Here's the drawing with two shaded views (mm, measured from the low corner). I have some questions. Round coordinates to 2 decimals unless told otherwise and drop trailing zeros. Order: outer loops, then holes, each group sorted by start corner. A loop starts at its lowest first (then second) coordinate and runs counter-clockwise, first axis right, second up. Notation, with made-up numbers: (56.25, 20) - (75.25, 20) arc R19 cw to (75.25, 26) - close; hole circle Ø3 at (4.25, 25). An arc over 180 degrees is marked (long way). Return JSON: item names as keys, results as strings. Group by question number.
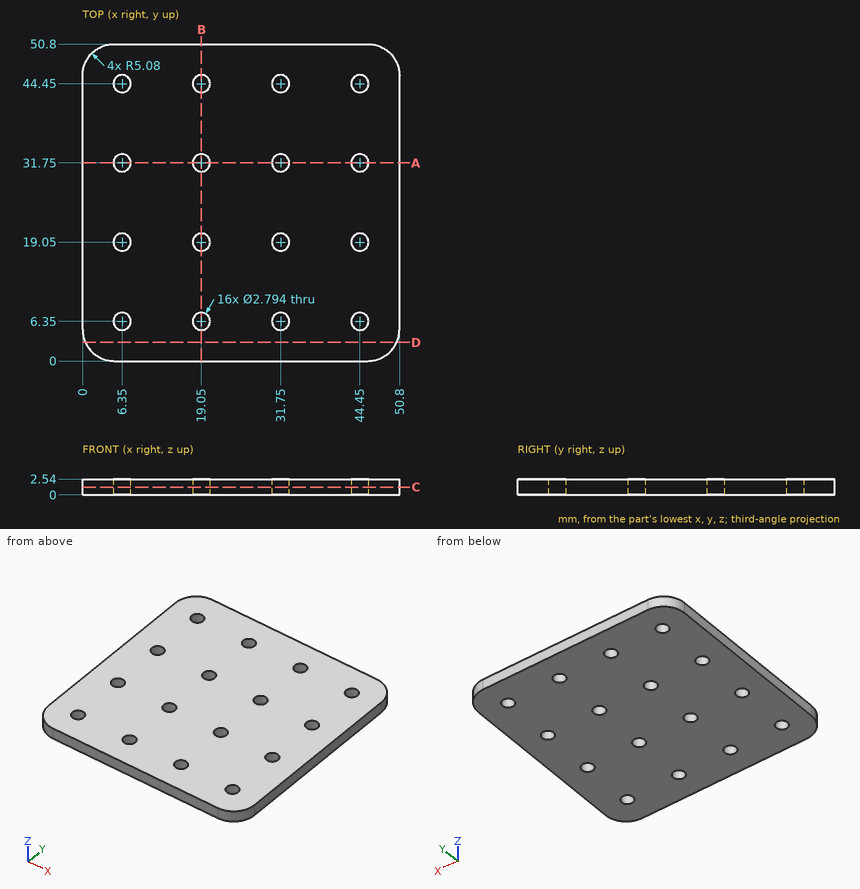
1) I want a section at A-A, the plane y = 31.75. List the corners of the cut face in (x, z) for me, plus the area to 3 significant figures.
2) I want a section at D-D, the plane y = 3. List the corners of the cut face in (x, z) for me.
3) Will this pin go through, and if not, where does the flat tip stop? pin 1 (3.5 mm diameter, centred on x = 6.35, y = 19.05, fed in from -Z).
4) I want a section at C-C, the plane z = 1.25. Give the number of separate pieces and of enclosed holes in the cut face, plus the area to 3 significant figures.
5) If I drill on line 1 along Y through (x, z) = (44.45, 1.15); line 2 along Y through (x, z) = (30.5, 2.2); line 3 along X through (y, z) = (18, 1.25), over which ranges is the centre line in solid material (lowest first)? Write a range as from..to.
Outcome:
{
 "1": {"outline": "(0, 0) - (4.95, 0) - (4.95, 2.54) - (0, 2.54) - close; (7.75, 0) - (17.65, 0) - (17.65, 2.54) - (7.75, 2.54) - close; (20.45, 0) - (30.35, 0) - (30.35, 2.54) - (20.45, 2.54) - close; (33.15, 0) - (43.05, 0) - (43.05, 2.54) - (33.15, 2.54) - close; (45.85, 0) - (50.8, 0) - (50.8, 2.54) - (45.85, 2.54) - close", "area": "101 mm^2"},
 "2": {"outline": "(0.45, 0) - (50.35, 0) - (50.35, 2.54) - (0.45, 2.54) - close"},
 "3": {"pin 1": "z = 0"},
 "4": {"separate pieces": "1", "enclosed holes": "16", "area": "2,460 mm^2"},
 "5": {"line 1": "0..4.95, 7.75..17.65, 20.45..30.35, 33.15..43.05, 45.85..50.8", "line 2": "0..5.73, 6.97..18.43, 19.67..31.13, 32.37..43.83, 45.07..50.8", "line 3": "0..5.43, 7.27..18.13, 19.97..30.83, 32.67..43.53, 45.37..50.8"}
}
